Here's how the part is built. I have some questions about the finished solid (model axes, mm). Coordinates: 2 decimals unless noted, no trailing zeros. Loops run counter-clockwise (first coordinate to the right, second up) from the corner with the lowest first, then second, coordinate; pieces in that order, holes last.
from build123d import *

# Parameters (mm, degrees)
SKETCH_1_W          = 6
SKETCH_1_H          = 60
SKETCH_1_R          = 1.55
EXTRUDE_1_DEPTH     = 2
CUT_EXTRUDE_1_DEPTH = 31.215889859


with BuildPart() as part:
    # ｽｹｯﾁ1 → ﾎﾞｽ - 押し出し1 (new body)
    with BuildSketch(Plane.XY):
        Rectangle(SKETCH_1_W, SKETCH_1_H)
        with Locations((0, 27)):
            Circle(SKETCH_1_R, mode=Mode.SUBTRACT)
        with Locations((0, -27)):
            Circle(SKETCH_1_R, mode=Mode.SUBTRACT)
    extrude(amount=EXTRUDE_1_DEPTH)

    # ｽｹｯﾁ2 → ｶｯﾄ - 押し出し1 (cut, through all)
    with BuildSketch(Plane.XY.offset(2)):
        with BuildLine():
            Line((-3, 12), (-3, -12))
            ThreePointArc((-3, -12), (1.583592135, 0), (-3, 12))
        make_face()
    extrude(amount=-CUT_EXTRUDE_1_DEPTH, mode=Mode.SUBTRACT)


solid = part.part
Q1. Suppose I cut it at D-D on x = 0.45. Write out the boundary of the cut face in (y, z), and give its area (3 significant figures).
Q2. We'd pull the mould along X, two halves only. Please class faces 1 (the flat face through (2, 0, 2)), 2 (the flat face through (-3, 21, 1)), 3 (the cylindrical face through (-0.202, -25.463, 0.986)), 4 (the cylindrical face through (-0.202, 28.537, 0.986)): pulls with the +X half, pulls with the -X half, needs draft (parallel to the pull), parting line crosses it, or undercut.
Q3. Will this pin go through, and if not, where does the flat tip stop? P1, Ø1.5, axis at x = -0.5, y = -8.5, coming from the -Z side.
Q4. Please list where these lines run through material, in increasing order: probe 1 along Y at (x, z) = (0.2, 0.8); probe 2 along Y at (x, z) = (0, 1.5); probe 3 along X at (y, z) = (26.5, 0.4).
Q5. Suppose I cut it at A-A on y = -27. Write out the boundary of the cut face in (x, z), and give its area (3 significant figures).
Q6. Suppose I cut it at B-B on z = 0.75. Write out the boundary of the cut face in (x, y).
Q7. Suppose I cut it at C-C on x = -2.4. Write out the boundary of the cut face in (y, z), and give its area (3 significant figures).
Check values:
1. outline: (-30, 0) - (-28.48, 0) - (-28.48, 2) - (-30, 2) - close; (-25.52, 0) - (-6.29, 0) - (-6.29, 2) - (-25.52, 2) - close; (6.29, 0) - (25.52, 0) - (25.52, 2) - (6.29, 2) - close; (28.48, 0) - (30, 0) - (30, 2) - (28.48, 2) - close
1. area: 83.0 mm2
2. face 1: needs draft
2. face 2: pulls with the -X half
2. face 3: undercut
2. face 4: undercut
3. P1: stops at z = 0
4. probe 1: y = -30 to -28.54, -25.46 to -6.92, 6.92 to 25.46, 28.54 to 30
4. probe 2: y = -30 to -28.55, -25.45 to -7.38, 7.38 to 25.45, 28.55 to 30
4. probe 3: x = -3 to -1.47, 1.47 to 3
5. outline: (-3, 0) - (-1.55, 0) - (-1.55, 2) - (-3, 2) - close; (1.55, 0) - (3, 0) - (3, 2) - (1.55, 2) - close
5. area: 5.80 mm2
6. outline: (-3, -30) - (3, -30) - (3, 30) - (-3, 30) - (-3, 12) arc R18 cw to (-3, -12) - close; hole circle Ø3.1 at (0, -27); hole circle Ø3.1 at (0, 27)
7. outline: (-30, 0) - (-11.29, 0) - (-11.29, 2) - (-30, 2) - close; (11.29, 0) - (30, 0) - (30, 2) - (11.29, 2) - close
7. area: 74.8 mm2
